Work out the finished part from the listing and answer in its coordinate system (mm). A direction names the side the tool comes from. Coordinates: 2 decimals unless noted, no trailing zeros. Order: outer loops, then holes, each group sorted by start corner. A loop starts at its lowest first (then second) coordinate and runs counter-clockwise, first axis right, second up. Notation, with made-up numbers: (54, 47) - (99, 47) arc R6 ccw to (99, 54) - close; hole circle Ø9 at (70.5, 77). An arc over 180 degrees is marked (long way). Answer as a JSON object with one key per item and string values. Group by question number.
1) Section B-B (x = 0) is taken. Give the vertices of the cut face in (y, z) (3 decimals), plus the area to 3 significant figures.
2) Section C-C (y = -23) is taken. Give the vertices of the cut face in (x, z) (1 decimal), plus the area to 3 significant figures.
3) Section A-A (z = 0) is taken. Give the vertices of the cut face in (x, y) (3 decimals), plus the area to 3 significant figures.
4) Section D-D (y = -13) is taken. Give the vertices of the cut face in (x, z) (1 decimal).
5) Each of these flat-tipped pins is pushed along its axis until it touches: P1, Ø4, axis at x = -21, y = -20, coming from the +Z side; P2, Ø3.5, axis at x = -7.88, z = 5.35, coming from the -Y side; P3, Ø4, axis at y = -4.5, z = 3.5, coming from the -X side. Where does it stop, or does it pass through?
6) A tool of negligible diameter and unlimited length cuts with its end or side. For faces 1 (the face through (-7.49, -20.74, -33.74)), 2 (the face through (-9.783, -17.887, 5.434)), 3 (the face through (-15.963, -2.504, -10.465)), from which of +Z, -Z, +X, -X, +Y, -Y can it reach the whole face along a straight path? Write none if from no direction.
7) The mould has two halves that part along X. Classify faces 4 (the face through (-7.49, -4.56, -33.74)), 5 (the face through (9.525, -2.504, -0.08)), 6 (the face through (7.716, -2.576, 6.435)), 7 (the face through (0, -25.4, 0)): released by +X, released by -X, zero draft, split by the parting line, or undercut.
8) Find the intervals of material crossed by line 1 along X through (y, z) = (-3.25, -8); line 2 along Y through (x, z) = (0, -14); line 3 along Z through (x, y) = (-3, -3), in increasing order.
from build123d import *

# Parameters (mm, degrees)
F0_R     = 34.561988
F1_DEPTH = 25.4
F3_DEPTH = 5.08
F4_R     = 1.27
F5_R     = 4.785324
F7_SIZE  = 2.54
F8_R     = 1.905
F9_DEPTH = 15.24


with BuildPart() as f1:
    # F0 (on Front) → F1 (new body)
    with BuildSketch(Plane.XZ):
        Circle(F0_R)
        with BuildLine():
            ThreePointArc((16.74505, -23.154566), (0, -28.575), (-16.74505, -23.154566))
            Line((-16.74505, -23.154566), (-5.581683, -7.718189))
            ThreePointArc((-5.581683, -7.718189), (0, -9.525), (5.581683, -7.718189))
            Line((5.581683, -7.718189), (16.74505, -23.154566))
        make_face(mode=Mode.SUBTRACT)
        with BuildLine():
            Line((-25.330056, 13.22569), (-7.497648, 5.874598))
            ThreePointArc((-7.497648, 5.874598), (-9.525, 0), (-7.497648, -5.874598))
            Line((-7.497648, -5.874598), (-25.330056, -13.22569))
            ThreePointArc((-25.330056, -13.22569), (-28.575, 0), (-25.330056, 13.22569))
        make_face(mode=Mode.SUBTRACT)
        with BuildLine():
            ThreePointArc((7.497648, -5.874598), (9.525, 0), (7.497648, 5.874598))
            Line((7.497648, 5.874598), (25.330056, 13.22569))
            ThreePointArc((25.330056, 13.22569), (28.575, 0), (25.330056, -13.22569))
            Line((25.330056, -13.22569), (7.497648, -5.874598))
        make_face(mode=Mode.SUBTRACT)
        with BuildLine():
            Line((-5.581683, 7.718189), (-16.74505, 23.154566))
            ThreePointArc((-16.74505, 23.154566), (0, 28.575), (16.74505, 23.154566))
            Line((16.74505, 23.154566), (5.581683, 7.718189))
            ThreePointArc((5.581683, 7.718189), (0, 9.525), (-5.581683, 7.718189))
        make_face(mode=Mode.SUBTRACT)
        with BuildLine():
            Line((25.330056, 13.22569), (7.497648, 5.874598))
            ThreePointArc((7.497648, 5.874598), (9.525, 0), (7.497648, -5.874598))
            Line((7.497648, -5.874598), (25.330056, -13.22569))
            ThreePointArc((25.330056, -13.22569), (28.575, 0), (25.330056, 13.22569))
        make_face()
        with BuildLine():
            ThreePointArc((16.74505, 23.154566), (0, 28.575), (-16.74505, 23.154566))
            Line((-16.74505, 23.154566), (-5.581683, 7.718189))
            ThreePointArc((-5.581683, 7.718189), (0, 9.525), (5.581683, 7.718189))
            Line((5.581683, 7.718189), (16.74505, 23.154566))
        make_face()
        with BuildLine():
            ThreePointArc((-7.497648, -5.874598), (-9.525, 0), (-7.497648, 5.874598))
            Line((-7.497648, 5.874598), (-25.330056, 13.22569))
            ThreePointArc((-25.330056, 13.22569), (-28.575, 0), (-25.330056, -13.22569))
            Line((-25.330056, -13.22569), (-7.497648, -5.874598))
        make_face()
        with BuildLine():
            Line((-5.581683, -7.718189), (-16.74505, -23.154566))
            ThreePointArc((-16.74505, -23.154566), (0, -28.575), (16.74505, -23.154566))
            Line((16.74505, -23.154566), (5.581683, -7.718189))
            ThreePointArc((5.581683, -7.718189), (0, -9.525), (-5.581683, -7.718189))
        make_face()
    extrude(amount=F1_DEPTH)

    # F2 (on face) → F3 (cut)
    with BuildSketch(Plane(origin=(0, 0, 0), x_dir=(-1, 0, 0), z_dir=(0, 1, 0))):
        with BuildLine():
            ThreePointArc((-6.894682, -6.571833), (-9.525, 0), (-6.894682, 6.571833))
            Line((-6.894682, 6.571833), (-24.770568, 14.246038))
            ThreePointArc((-24.770568, 14.246038), (-28.575, 0), (-24.770568, -14.246038))
            Line((-24.770568, -14.246038), (-6.894682, -6.571833))
        make_face()
        with BuildLine():
            Line((-15.190351, 24.202972), (-5.06345, 8.067657))
            ThreePointArc((-5.06345, 8.067657), (0, 9.525), (5.06345, 8.067657))
            Line((5.06345, 8.067657), (15.190351, 24.202972))
            ThreePointArc((15.190351, 24.202972), (0, 28.575), (-15.190351, 24.202972))
        make_face()
        with BuildLine():
            Line((24.770568, 14.246038), (6.894682, 6.571833))
            ThreePointArc((6.894682, 6.571833), (9.525, 0), (6.894682, -6.571833))
            Line((6.894682, -6.571833), (24.770568, -14.246038))
            ThreePointArc((24.770568, -14.246038), (28.575, 0), (24.770568, 14.246038))
        make_face()
        with BuildLine():
            ThreePointArc((5.06345, -8.067657), (0, -9.525), (-5.06345, -8.067657))
            Line((-5.06345, -8.067657), (-15.190351, -24.202972))
            ThreePointArc((-15.190351, -24.202972), (0, -28.575), (15.190351, -24.202972))
            Line((15.190351, -24.202972), (5.06345, -8.067657))
        make_face()
    extrude(amount=-F3_DEPTH, mode=Mode.SUBTRACT)

    # F4
    f4_edges = [f1.edges().sort_by_distance(p)[0] for p in [
        (24.770568, -2.54, 14.246038),
        (24.770568, -2.54, -14.246038),
        (6.894682, -2.54, -6.571833),
        (6.894682, -2.54, 6.571833),
        (5.06345, -2.54, 8.067657),
        (15.190351, -2.54, 24.202972),
        (-15.190351, -2.54, 24.202972),
        (-5.06345, -2.54, 8.067657),
        (-6.894682, -2.54, 6.571833),
        (-6.894682, -2.54, -6.571833),
        (-24.770568, -2.54, -14.246038),
        (-24.770568, -2.54, 14.246038),
        (-5.06345, -2.54, -8.067657),
        (5.06345, -2.54, -8.067657),
        (15.190351, -2.54, -24.202972),
        (-15.190351, -2.54, -24.202972),
    ]]
    fillet(f4_edges, radius=F4_R)

    # F5 (on Top) → F6 (revolve, cut)
    with BuildSketch(Plane.XY):
        with Locations((34.664739, -11.4271)):
            Circle(F5_R)
    revolve(axis=Axis((0, 0, 0), (0, 1, 0)), mode=Mode.SUBTRACT)

    # F7
    f7_edges = [f1.edges().sort_by_distance(p)[0] for p in [
        (-34.561988, 0, 0),
    ]]
    chamfer(f7_edges, length=F7_SIZE)

    # F8 (on face) → F9 (cut)
    with BuildSketch(Plane.XZ.offset(25.4)):
        with Locations((-7.88021, 5.350506)):
            Circle(F8_R)
        with Locations((7.88021, 5.350506)):
            Circle(F8_R)
        with Locations((0, -9.525)):
            Circle(F8_R)
    extrude(amount=-F9_DEPTH, mode=Mode.SUBTRACT)


solid = f1.part
Report:
{
 "1": {"outline": "(-25.4, -34.562) - (-16.211, -34.562) arc R4.785 cw to (-6.643, -34.562) - (-2.54, -34.562) - (0, -32.022) - (0, -28.575) - (-5.08, -28.575) - (-5.08, -9.525) - (0, -9.525) - (0, 9.525) - (-5.08, 9.525) - (-5.08, 28.575) - (0, 28.575) - (0, 32.022) - (-2.54, 34.562) - (-6.643, 34.562) arc R4.785 cw to (-16.211, 34.562) - (-25.4, 34.562) - (-25.4, -7.62) - (-10.16, -7.62) - (-10.16, -11.43) - (-25.4, -11.43) - close", "area": "1,430 mm²"},
 "2": {"outline": "circle Ø69.1 at (0, 0); hole circle Ø3.8 at (-7.9, 5.4); hole circle Ø3.8 at (0, -9.5); hole circle Ø3.8 at (7.9, 5.4)", "area": "3,720 mm²"},
 "3": {"outline": "(-34.562, -25.4) - (34.562, -25.4) - (34.562, -16.211) arc R4.785 cw to (34.562, -6.643) - (34.562, -2.54) - (32.022, 0) - (28.575, 0) - (28.575, -5.08) - (9.525, -5.08) - (9.525, 0) - (-9.525, 0) - (-9.525, -5.08) - (-28.575, -5.08) - (-28.575, 0) - (-32.022, 0) - (-34.562, -2.54) - (-34.562, -6.643) arc R4.785 cw to (-34.562, -16.211) - close", "area": "1,490 mm²"},
 "4": {"outline": "circle Ø60.3 at (0, 0); hole circle Ø3.8 at (-7.9, 5.4); hole circle Ø3.8 at (0, -9.5); hole circle Ø3.8 at (7.9, 5.4)"},
 "5": {"P1": "stops at z = 28.87", "P2": "stops at y = -10.16", "P3": "stops at x = -34.53"},
 "6": {"face 1": "+Y, -Y", "face 2": "-Y", "face 3": "+Y"},
 "7": {"face 4": "split by the parting line", "face 5": "undercut", "face 6": "undercut", "face 7": "zero draft"},
 "8": {"line 1": "x = -33.62 to -27.43, -10.22 to 10.22, 27.43 to 33.62", "line 2": "y = -25.4 to -5.08", "line 3": "z = -34.43 to -28.42, -9.04 to 9.04, 28.42 to 34.43"}
}
